from build123d import *


with BuildPart() as f1:
    # F0 (on Front) → F1 (revolve)
    with BuildSketch(Plane.XZ):
        with BuildLine():
            Line((3.25, 16), (3.25, 0))
            Line((3.25, 0), (6.75, 0))
            Line((6.75, 0), (6.75, 1))
            Line((6.75, 1), (5.25, 1))
            Line((5.25, 1), (5.25, 3))
            ThreePointArc((5.25, 3), (10.245024, 8.002927), (5.25, 13.005855))
            Line((5.25, 13.005855), (5.25, 15))
            Line((5.25, 15), (6.75, 15))
            Line((6.75, 15), (6.75, 16))
            Line((6.75, 16), (3.25, 16))
        make_face()
    revolve(axis=Axis((0, 0, 15.346395), (0, 0, 1)))


solid = f1.part
For this review, take the finished solid that the model builds, in its own axes (mm). A direction names the side the tool comes from. Round coordinates to 2 decimals unless told otherwise and drop trailing zeros. Order: outer loops, then holes, each group sorted by start corner. A loop starts at its lowest first (then second) coordinate and runs counter-clockwise, first axis right, second up. Notation, with made-up numbers: M 12,62 L 70,62 A8 ccw 70,67 Z; hole C -6.5,-38.5 d1. An arc over 180 degrees is marked long. Use a Markdown table: item, result. Add a question column.
Item 1: Add section C-C, the plane z = 13.75. Give the boundary of the cut face in (x, y), then the cut area to 3 significant figures.
Item 2: To check wall thickness, follow line 1 along Z through (x, y) = (-6.25, -0.75); line 2 along Z through (x, y) = (4.75, -3.25); line 3 along Y through (x, z) = (0, 7.25). State the ranges of each line that lie inside material, in increasing order.
Item 3: Insertion check: pin 1 (8 mm diameter, centred on x = 5, z = 3, fed in from +Y); pin 2 (8 mm diameter, centred on x = -2, z = 14, fed in from +Y); pin 3 (6 mm diameter, centred on y = 8, z = 6.5, fed in from +X). Each pin has a flat end and moves straight along its axis. Give the tip position at first contact, or say it passes through.
Item 4: Mouldability with a two-part tool opening along X and no side actions: class faces 4 (the cylindrical face through (-2.579, -1.978, 7.888)), 5 (the cylindrical face through (5, 1.6, 2)), 6 (the flat face through (0, -5.5, 15)) as released by +X, released by -X, zero draft, split by the parting line, or undercut.
Item 5: Tool access review of faces 1 (the cylindrical face through (-1.46, -6.59, 0.51)), 2 (the cylindrical face through (-1.46, -6.59, 15.51)), 3 (the flat face through (0, -5.5, 1)): name each direction out of +Z, -Z, +X, -X, +Y, -Y from which nothing blocks a thin tool from reaching the whole face with its end or side.
Item 6: Add section A-A, the plane x = 0. Give the boundary of the cut face in (y, z).
Item 7: Add section D-D, the plane x = 6. State how many separate pieces and enclosed holes the cut face has, then the cut area to 3 significant figures.
Geometry results:
| question | item | result |
|---|---|---|
| 1 | outline | C 0,0 d10.5; hole C 0,0 d6.5 |
| 1 | area | 53.4 mm² |
| 2 | line 1 | z = 0 to 1, 3.11 to 12.89, 15 to 16 |
| 2 | line 2 | z = 0 to 1, 3.03 to 12.98, 15 to 16 |
| 2 | line 3 | y = -10.19 to -3.25, 3.25 to 10.19 |
| 3 | pin 1 | stops at y = 9.56 |
| 3 | pin 2 | stops at y = 9.72 |
| 3 | pin 3 | stops at x = 8.82 |
| 4 | face 4 | undercut |
| 4 | face 5 | split by the parting line |
| 4 | face 6 | zero draft |
| 5 | face 1 | -Z |
| 5 | face 2 | +Z |
| 5 | face 3 | none |
| 6 | outline | M -6.75,0 L -3.25,0 L -3.25,16 L -6.75,16 L -6.75,15 L -5.25,15 L -5.25,13.01 A5 ccw -5.25,3 L -5.25,1 L -6.75,1 Z; M 3.25,0 L 6.75,0 L 6.75,1 L 5.25,1 L 5.25,3 A5 ccw 5.25,13.01 L 5.25,15 L 6.75,15 L 6.75,16 L 3.25,16 Z |
| 7 | separate pieces | 3 |
| 7 | enclosed holes | 0 |
| 7 | area | 149 mm² |
